Model file for the job. Use its own axes, mm. Coordinates: 2 decimals unless noted, no trailing zeros. Write each loop counter-clockwise with the first axis right and the second up, starting at its lowest first coordinate (ties: lowest second). Pieces come first, ordered by that corner, then holes. Notation, with made-up numbers: (78, -17.75) -> (84, -17.75) arc R20 ccw to (84, 6.25) -> close; hole circle Ø5 at (74, 10). An arc over 180 degrees is marked (long way). Answer as a JSON object with one key per item and string values. Group by question number.
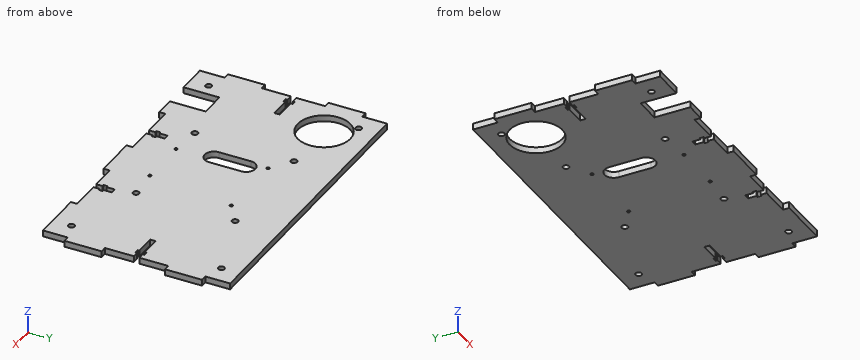
from build123d import *

# Parameters (mm, degrees)
SKETCH1_W           = 240
SKETCH1_H           = 151
BOSS_EXTRUDE1_DEPTH = 5
SKETCH2_R           = 1.25
CUT_EXTRUDE1_DEPTH  = 5
CUT_EXTRUDE2_DEPTH  = 10
SKETCH6_R           = 2.5
CUT_EXTRUDE3_DEPTH  = 10
SKETCH7_R           = 2.5
CUT_EXTRUDE4_DEPTH  = 10
SKETCH8_W           = 21.1
SKETCH8_H           = 29
CUT_EXTRUDE5_DEPTH  = 10
SKETCH9_W           = 5
SKETCH9_H           = 30
BOSS_EXTRUDE2_DEPTH = 5
CUT_EXTRUDE6_DEPTH  = 5
SKETCH11_W          = 50
SKETCH11_H          = 5
SKETCH11_W_2        = 50.1
CUT_EXTRUDE7_DEPTH  = 10
CUT_EXTRUDE8_DEPTH  = 10
SKETCH15_R          = 21.25
CUT_EXTRUDE9_DEPTH  = 10


with BuildPart() as part:
    # Sketch1 → Boss-Extrude1 (new body)
    with BuildSketch(Plane.XY):
        Rectangle(SKETCH1_W, SKETCH1_H)
    extrude(amount=BOSS_EXTRUDE1_DEPTH)

    # Sketch2 → Cut-Extrude1 (cut)
    with BuildSketch(Plane(origin=(0, 0, 0), x_dir=(-1, 0, 0), z_dir=(0, 0, -1))):
        with Locations((28, 28)):
            Circle(SKETCH2_R)
        with Locations((-28, 28)):
            Circle(SKETCH2_R)
        with Locations((20, -42)):
            Circle(SKETCH2_R)
        with Locations((-20, -42)):
            Circle(SKETCH2_R)
    extrude(amount=-CUT_EXTRUDE1_DEPTH, mode=Mode.SUBTRACT)

    # Sketch5 → Cut-Extrude2 (cut)
    with BuildSketch(Plane(origin=(0, 0, 0), x_dir=(-1, 0, 0), z_dir=(0, 0, -1))):
        with BuildLine():
            Line((15.5, -13), (15.5, 13))
            ThreePointArc((15.5, 13), (23, 20.5), (30.5, 13))
            Line((30.5, 13), (30.5, -13))
            ThreePointArc((30.5, -13), (23, -20.5), (15.5, -13))
        make_face()
    extrude(amount=-CUT_EXTRUDE2_DEPTH, mode=Mode.SUBTRACT)

    # Sketch6 → Cut-Extrude3 (cut)
    with BuildSketch(Plane(origin=(0, 0, 0), x_dir=(-1, 0, 0), z_dir=(0, 0, -1))):
        with Locations((-105, 60.5)):
            Circle(SKETCH6_R)
        with Locations((-105, -60.5)):
            Circle(SKETCH6_R)
        with Locations((105, -60.5)):
            Circle(SKETCH6_R)
        with Locations((105, 60.5)):
            Circle(SKETCH6_R)
    extrude(amount=-CUT_EXTRUDE3_DEPTH, mode=Mode.SUBTRACT)

    # Sketch7 → Cut-Extrude4 (cut)
    with BuildSketch(Plane(origin=(0, 0, 0), x_dir=(-1, 0, 0), z_dir=(0, 0, -1))):
        with Locations((45, 40)):
            Circle(SKETCH7_R)
        with Locations((45, -40)):
            Circle(SKETCH7_R)
        with Locations((-45, 40)):
            Circle(SKETCH7_R)
        with Locations((-45, -40)):
            Circle(SKETCH7_R)
    extrude(amount=-CUT_EXTRUDE4_DEPTH, mode=Mode.SUBTRACT)

    # Sketch8 → Cut-Extrude5 (cut)
    with BuildSketch(Plane(origin=(0, 0, 0), x_dir=(-1, 0, 0), z_dir=(0, 0, -1))):
        with Locations((84.45, -61)):
            Rectangle(SKETCH8_W, SKETCH8_H)
    extrude(amount=-CUT_EXTRUDE5_DEPTH, mode=Mode.SUBTRACT)

    # Sketch9 → Boss-Extrude2 (add)
    with BuildSketch(Plane(origin=(0, 0, 0), x_dir=(-1, 0, 0), z_dir=(0, 0, -1))):
        with Locations((122.5, 40.5)):
            Rectangle(SKETCH9_W, SKETCH9_H)
        with Locations((122.5, -40.5)):
            Rectangle(SKETCH9_W, SKETCH9_H)
        with Locations((-122.5, -40.5)):
            Rectangle(SKETCH9_W, SKETCH9_H)
        with Locations((-122.5, 40.5)):
            Rectangle(SKETCH9_W, SKETCH9_H)
    extrude(amount=-BOSS_EXTRUDE2_DEPTH)

    # Sketch10 → Cut-Extrude6 (cut)
    with BuildSketch(Plane(origin=(0, 0, 0), x_dir=(-1, 0, 0), z_dir=(0, 0, -1))):
        Polygon((-120, 2.2), (-115, 2.2), (-115, 3.7), (-111.7, 3.7), (-111.7, 2.2), (-95, 2.2), (-95, -2.2), (-111.7, -2.2), (-111.7, -3.7), (-115, -3.7), (-115, -2.2), (-120, -2.2), align=None)
        Polygon((115, -2.2), (120, -2.2), (120, 2.2), (115, 2.2), (115, 3.7), (111.7, 3.7), (111.7, 2.2), (95, 2.2), (95, -2.2), (111.7, -2.2), (111.7, -3.7), (115, -3.7), align=None)
    extrude(amount=-CUT_EXTRUDE6_DEPTH, mode=Mode.SUBTRACT)

    # Sketch11 → Cut-Extrude7 (cut)
    with BuildSketch(Plane(origin=(0, 0, 0), x_dir=(-1, 0, 0), z_dir=(0, 0, -1))):
        with Locations((32.75, -73)):
            Rectangle(SKETCH11_W, SKETCH11_H)
        with Locations((-52.3, -73)):
            Rectangle(SKETCH11_W_2, SKETCH11_H)
    extrude(amount=-CUT_EXTRUDE7_DEPTH, mode=Mode.SUBTRACT)

    # Sketch12 → Cut-Extrude8 (cut)
    with BuildSketch(Plane(origin=(0, 0, 0), x_dir=(-1, 0, 0), z_dir=(0, 0, -1))):
        Polygon((-52.35, -55.5), (-52.35, -62.2), (-53.85, -62.2), (-53.85, -65.5), (-52.35, -65.5), (-52.35, -70.5), (-47.95, -70.5), (-47.95, -65.5), (-46.45, -65.5), (-46.45, -62.2), (-47.95, -62.2), (-47.95, -55.5), align=None)
        Polygon((32.85, -70.5), (28.45, -70.5), (28.45, -65.5), (26.95, -65.5), (26.95, -62.2), (28.45, -62.2), (28.45, -55.5), (32.85, -55.5), (32.85, -62.2), (34.35, -62.2), (34.35, -65.5), (32.85, -65.5), align=None)
    extrude(amount=-CUT_EXTRUDE8_DEPTH, mode=Mode.SUBTRACT)

    # Sketch15 → Cut-Extrude9 (cut)
    with BuildSketch(Plane(origin=(0, 0, 0), x_dir=(-1, 0, 0), z_dir=(0, 0, -1))):
        with Locations((90, 40.5)):
            Circle(SKETCH15_R)
    extrude(amount=-CUT_EXTRUDE9_DEPTH, mode=Mode.SUBTRACT)


solid = part.part
(1) Cut at C-C on x = -77. List the corners of the cut face in (y, z), plus the area to 3 significant figures.
(2) Pin check, flat tips, straight feed: pin 1 (1.5 mm diameter, centred on x = 74, y = -27.5, fed in from -Z); pin 2 (1 mm diameter, centred on y = 12, z = 4, fed in from -X); pin 3 (1.6 mm diameter, centred on x = -33.5, z = 1.5, fed in from -Y); pin 4 (2.5 mm diameter, centred on x = -122, z = 3, fed in from +Y). Stop position of each tip, or through.
(3) Cut at A-A on x = -45. List the corners of the cut face in (y, z), plus the area to 3 significant figures.
(4) Cut at D-D on z = 4.1. Give the number of separate pieces and of enclosed holes in the cut face, plus the area to 3 significant figures.
(5) Wall check: probe 1 along Y at (x, z) = (105, 3.3); probe 2 along Y at (x, z) = (-45, 1.35); probe 3 along X at (y, z) = (2.5, 1.15). Give the ranges that are in metal, low to high.
(6) Cut at B-B on x = 105. List the corners of the cut face in (y, z), plus the area to 3 significant figures.
Results found:
{
 "1": {"outline": "(-46.5, 0) -> (23.69, 0) -> (23.69, 5) -> (-46.5, 5) -> close; (57.31, 0) -> (75.5, 0) -> (75.5, 5) -> (57.31, 5) -> close", "area": "442 mm²"},
 "2": {"pin 1": "stops at z = 0", "pin 2": "stops at x = -120", "pin 3": "stops at y = -70.5", "pin 4": "stops at y = 55.5"},
 "3": {"outline": "(-70.5, 0) -> (-42.5, 0) -> (-42.5, 5) -> (-70.5, 5) -> close; (-37.5, 0) -> (37.5, 0) -> (37.5, 5) -> (-37.5, 5) -> close; (42.5, 0) -> (75.5, 0) -> (75.5, 5) -> (42.5, 5) -> close", "area": "680 mm²"},
 "4": {"separate pieces": "1", "enclosed holes": "14", "area": "33,200 mm²"},
 "5": {"probe 1": "y = -75.5 to -63, -58 to -2.2, 2.2 to 58, 63 to 75.5", "probe 2": "y = -70.5 to -42.5, -37.5 to 37.5, 42.5 to 75.5", "probe 3": "x = -120 to -115, -111.7 to -30.5, -15.5 to 111.7, 115 to 120"},
 "6": {"outline": "(-75.5, 0) -> (-63, 0) -> (-63, 5) -> (-75.5, 5) -> close; (-58, 0) -> (-2.2, 0) -> (-2.2, 5) -> (-58, 5) -> close; (2.2, 0) -> (58, 0) -> (58, 5) -> (2.2, 5) -> close; (63, 0) -> (75.5, 0) -> (75.5, 5) -> (63, 5) -> close", "area": "683 mm²"}
}
